Check sheet for the modelled part. Datum: model origin and axes. Units: mm. A direction names the side the tool comes from. Give positions to 0.01 mm unless a question says otherwise; leave off trailing zeros. Order: outer loops, then holes, each group sorted by start corner. A loop starts at its lowest first (then second) coordinate and runs counter-clockwise, first axis right, second up. Notation, with made-up numbers: M 62,25.5 L 78,25.5 A27 cw 78,41.5 Z; hole C -36,31 d7. An arc over 180 degrees is marked long. Return JSON: item names as keys, results as strings. Group by question number.
Autodesk Inventor part; units mm, degrees
ref_plane "YZ Plane" through (0, 0, 0) normal (1, 0, 0) x (0, 1, 0)
ref_plane "XZ Plane" through (0, 0, 0) normal (0, 1, 0) x (-1, 0, 0)
ref_plane "XY Plane" through (0, 0, 0) normal (0, 0, 1) x (1, 0, 0)
sketch "Sketch1" plane through (0, 0, 0) normal (1, 0, 0) x (0, 1, 0)
  point P0 (0, 0)
sketch "Sketch2" plane through (0, 0, 0) normal (1, 0, 0) x (0, 1, 0)
  line L0 (32, 8.5828) -> (0, 8.5828)
  line L1 (0, 8.5828) -> (0, -31.4172)
  line L2 (0, -31.4172) -> (32, -31.4172)
  line L3 (32, -31.4172) -> (32, 8.5828)
  point P0 (0, 0)
  dimension "d0" = 32
  dimension "d1" = 40
extrude "Extrusion1" add sketch "Sketch2" along normal blind 10
sketch "Sketch3" plane through (10, 0, 0) normal (1, 0, 0) x (0, 0, -1)
  point P0 (0, 0)
sketch "Sketch4" plane through (10, 0, 0) normal (1, 0, 0) x (0, 0, -1)
  line L0 (-8.5828, 32) -> (-8.5828, 0)
  line L1 (-8.5828, 0) -> (31.4172, 0)
  line L2 (-8.5828, 32) -> (7.4172, 32)
  line L3 (7.4172, 32) -> (7.4172, 0)
  line L4 (7.4172, 0) -> (-8.5828, 0)
  line L5 (-8.5828, 0) -> (-8.5828, 32)
  point P0 (0, 0)
  dimension "d4" = 16
extrude "Extrusion2" add sketch "Sketch4" along normal blind 8
sketch "Sketch5" plane through (18, 0, 0) normal (1, 0, 0) x (0, 0, -1)
  line L0 (-8.5828, 32) -> (-8.5828, 0)
  line L1 (-8.5828, 0) -> (31.4172, 0)
  line L2 (-8.5828, 20) -> (7.4172, 20)
  line L3 (7.4172, 20) -> (7.4172, 0)
  line L4 (7.4172, 0) -> (-8.5828, 0)
  line L5 (-8.5828, 0) -> (-8.5828, 20)
  point P0 (0, 0)
  dimension "d7" = 16
  dimension "d8" = 20
extrude "Extrusion3" add sketch "Sketch5" along normal blind 19
properties part number "lab1ex1"
1) Sectioned sample at D-D on z = -19.5. Record the boundary of the cut face in (x, y), then the cut area to 3 significant figures.
2) Material ranges on line 1 along Z through (x, y) = (17, 21.5); line 2 along X through (y, z) = (9.5, -9); line 3 along X through (y, z) = (24.5, 0.5), recorded low to high.
3) Sectioned sample at A-A on z = 5. Record the boundary of the cut face in (x, y), then the cut area to 3 significant figures.
4) Tool access check on faces 1 (the face through (7, 32, -7)), 2 (the face through (10, 16, -19)), 3 (the face through (18, 26, 1)). Record the directions out of +Z, -Z, +X, -X, +Y, -Y that give a thin tool (end or side, any length) a straight path to the whole face; none if there is none.
5) Depth check by flat-ended pin: P1, Ø12, axis at y = 12.5, z = -23, coming from the +X side; P2, Ø8, axis at x = 23.5, y = 15, coming from the -Z side; P3, Ø13, axis at y = 28, z = 0.5, coming from the +X side. Enter the tip coordinate at first touch or a pass-through.
6) Sectioned sample at B-B on y = 14. Record the boundary of the cut face in (x, z).
7) Sectioned sample at C-C on x = 32. Record the boundary of the cut face in (y, z), then the cut area to 3 significant figures.
Reply:
{
 "1": {"outline": "M 0,0 L 10,0 L 10,32 L 0,32 Z", "area": "320 mm^2"},
 "2": {"line 1": "-7.42 to 8.58", "line 2": "0 to 10", "line 3": "0 to 18"},
 "3": {"outline": "M 0,0 L 37,0 L 37,20 L 18,20 L 18,32 L 0,32 Z", "area": "956 mm^2"},
 "4": {"face 1": "+Z, -Z, +X, -X, +Y", "face 2": "-Z, +X, +Y, -Y", "face 3": "+Z, -Z, +X, +Y"},
 "5": {"P1": "x = 10", "P2": "z = -7.42", "P3": "x = 18"},
 "6": {"outline": "M 0,-31.42 L 10,-31.42 L 10,-7.42 L 37,-7.42 L 37,8.58 L 0,8.58 Z"},
 "7": {"outline": "M 0,-7.42 L 20,-7.42 L 20,8.58 L 0,8.58 Z", "area": "320 mm^2"}
}
